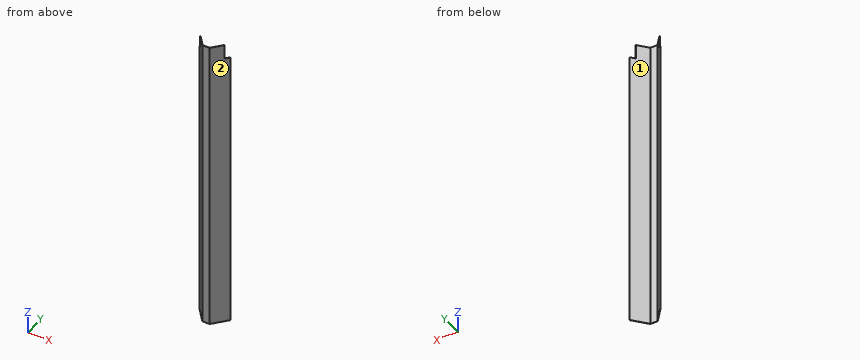
Autodesk Inventor part; units mm, degrees
ref_plane "YZ Plane" through (0, 0, 0) normal (1, 0, 0) x (0, 1, 0)
ref_plane "XZ Plane" through (0, 0, 0) normal (0, 1, 0) x (-1, 0, 0)
ref_plane "XY Plane" through (0, 0, 0) normal (0, 0, 1) x (1, 0, 0)
sketch "Sketch4" plane through (0, 0, 0) normal (0, 0, 1) x (1, 0, 0)
  line L0 (-25, 0) -> (-24.0674, 0) construction
  line L1 (25, 0) -> (25.5995, 0.7144) construction
  line L2 (-25, 0) -> (-25.5995, 0.7144) construction
  line L3 (-108.91, 100) -> (108.91, 100) construction
  arc A0 (-25.5995, 0.7144) -> (-24.0674, 0) centre (-24.0674, 2) ccw
  arc A1 (24.0674, 0) -> (25.5995, 0.7144) centre (24.0674, 2) ccw
  line L4 (24.0674, 0) -> (25, 0) construction
  line L5 (25.5995, 0.7144) -> (108.91, 100)
  line L6 (-25.5995, 0.7144) -> (-108.91, 100)
  line L7 (-24.0674, 0) -> (24.0674, 0)
  point P0 (0, 0)
  point P1 (0, 0)
  point P2 (0, 100)
  point P3 (0, 0)
  dimension "d14" = 217.8199
  dimension "d15" = 50
  dimension "d16" = 100
  dimension "d17" = 2
  dimension "d39" = 130
contour flange "Contour Flange2" sketch "Sketch4" thickness 2 bend radius 2 width 2050 along (0, 0, -1) mid plane no both sides no wall seen from (-67.2547, 50.3572, 0) lies toward (-0.7660444, -0.6427876, 0) curves L6 A0 L7 A1 L5
bend "Bend4"
corner "Corner4"
sketch "Sketch6" plane through (0, 0, 0) normal (1, 0, 0) x (0, 1, 0)
  line L0 (100, -2050) -> (100, 0)
  line L1 (-0.5712, 0) -> (98.7144, 0)
  line L2 (98.7144, 0) -> (98.7144, -2050)
  line L3 (98.7144, 0) -> (100, 0)
  line L4 (70, 0) -> (70, -100)
  line L5 (70, -100) -> (100, -100)
  point P0 (0, 0)
  dimension "d51" = 30
  dimension "d52" = 100
extrude "Extrusion1" cut sketch "Sketch6" along normal through all both and the other way through all
equation "\"d15\" = Лоток_ширина_низ"
equation "\"d16\" = Лоток_высота"
equation "\"d17\" = BendRadius"
equation "\"d39\" = Лоток_угол"
equation "\"d51\" = Лоток_глубина_выреза"
equation "\"d40\" = Thickness"
equation "\"d41\" = BendReliefWidth"
equation "\"d42\" = BendReliefDepth"
equation "\"d43\" = MinimumRemnant"
equation "\"d44\" = TransitionRadius"
equation "\"d46\" = BendRadius"
equation "\"d48\" = CornerReliefSize"
equation "\"d49\" = GapSize"
equation "\"d50\" = JacobiRadiusSize"
equation "\"BendRadius\" = Thickness"
equation "\"BendReliefWidth\" = Thickness"
equation "\"BendReliefDepth\" = 0.5 * Thickness"
equation "\"CornerReliefSize\" = 4 * Thickness"
equation "\"MinimumRemnant\" = 2 * Thickness"
equation "\"TransitionRadius\" = BendRadius"
equation "\"JacobiRadiusSize\" = BendRadius"
equation "\"GapSize\" = Thickness"
equation "\"Лоток_ширина_низ\" = 50"
equation "\"Лоток_высота\" = 100"
equation "\"Лоток_угол\" = 130deg"
equation "\"Лоток_глубина_выреза\" = 30"
properties part number "ДМФ 051 лоток илоотвод"
Check sheet for the modelled part. Datum: model origin and axes. Units: mm. Face numbers are marked on the shaded views. A direction names the side the tool comes from. Round coordinates to 2 decimals unless told otherwise and drop trailing zeros. Loops run counter-clockwise (first coordinate to the right, second up) from the corner with the lowest first, then second, coordinate; pieces in that order, holes last. Notation, with made-up numbers: M 9.25,71 L 64.25,71 A13 ccw 64.25,85 Z; hole C 27,2 d6. An arc over 180 degrees is marked long. One line per item, written item: value.
(1) Sectioned sample at B-B, the plane z = -1750. Record the cut outline in (x, y), then the cut area to 3 significant figures.
Computed values:
outline: M -110.44,98.71 L -27.13,-0.57 A4 ccw -24.07,-2 L 24.07,-2 A4 ccw 27.13,-0.57 L 110.44,98.71 L 108.91,100 L 25.6,0.71 A2 cw 24.07,0 L -24.07,0 A2 cw -25.6,0.71 L -108.91,100 Z
area: 625 mm^2
(2) Access from +Z, -Z, +X, -X, +Y, -Y to the whole of each face (thin tool, end or side, straight path). Record for the marked faces 1 and 2.
Computed values:
face 1: +Z, -Z, +Y
face 2: +Z, -Z, +X, -Y
(3) Depth check by flat-ended pin: pin 1 Ø5 at (x, z) = (39, -1679) entering from -Y; pin 2 Ø2 at (x, z) = (85, -57.5) entering from +Y; pin 3 Ø3 at (x, z) = (-56, -331) entering from +Y. Enter the tip coordinate at first touch or a pass-through.
Computed values:
pin 1: stops at y = 10.59
pin 2: stops at y = 70
pin 3: stops at y = 38.73
(4) Sectioned sample at A-A, the plane y = 19. Record the cut outline in (x, z).
Computed values:
outline: M -43.55,-2050 L -40.94,-2050 L -40.94,0 L -43.55,0 Z; M 40.94,-2050 L 43.55,-2050 L 43.55,0 L 40.94,0 Z
(5) Thickness scan on line 1 (Y direction, x = -10, z = -427); line 2 (X direction, y = 64, z = -1478.5); line 3 (X direction, y = 73.5, z = -421). Record the ranges inside material, lowest first.
Computed values:
line 1: y = -2 to 0
line 2: x = -81.31 to -78.7, 78.7 to 81.31
line 3: x = -89.28 to -86.67, 86.67 to 89.28
